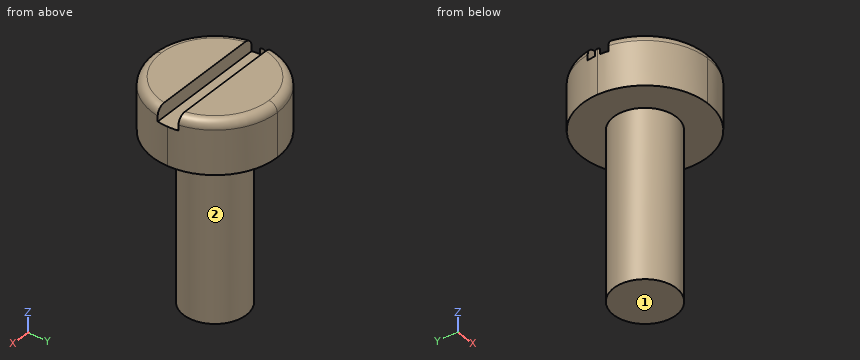
from build123d import *

# Parameters (mm, degrees)
F1_DEPTH    = 3.81
F2_T1_DEPTH = 22.225
F3_R        = 3.80999
F0_W        = 1.905
F0_H        = 10.16
F5_R        = 0.508
F7_DEPTH    = 0.8382


# Not quite as in the source:
# - a fillet or chamfer that OpenCascade refuses, or shapes differently, is made with other operations: its cross-section is extruded or revolved along the edge and cut away or added
# - a fillet or chamfer is up to 0.001 mm smaller than in the source, because OpenCascade refuses the exact size
# - ends of sketch curves that miss each other by under 0.0002 mm in the source are joined
# - a feature names something its author has since deleted; it is built from what else it names


with BuildPart() as f1:
    # F0 (on Front) → F1 (new body, symmetric)
    with BuildSketch(Plane.XZ):
        Polygon((-3.81, 3.175), (-3.81, 0), (-1.905, 0), (0, 0), (1.905, 0), (3.81, 0), (3.81, 3.175), align=None)
    extrude(amount=F1_DEPTH, both=True)

    # F2: fillet of radius 3.81 on 2 edges, made by hand

    # F2_s2 → F2_t1 (cut)
    with BuildSketch(Plane.XY.offset(-9.525)):
        with BuildLine():
            ThreePointArc((-3.81, 0), (-2.6940768363, -2.6940768363), (0, -3.81))
            Line((0, -3.81), (-3.81, -3.81))
            Line((-3.81, -3.81), (-3.81, 0))
        make_face()
        with BuildLine():
            ThreePointArc((-3.81, 0), (-2.6940768363, 2.6940768363), (0, 3.81))
            Line((0, 3.81), (-3.81, 3.81))
            Line((-3.81, 3.81), (-3.81, 0))
        make_face()
    extrude(amount=F2_T1_DEPTH, mode=Mode.SUBTRACT)

    # F3 (radius 3.81 in the source; OpenCascade refuses exactly that, so slightly less here)
    f3_edges = [f1.edges().sort_by_distance(p)[0] for p in [
        (3.81, -3.81, 1.5875),
        (3.81, 3.81, 1.5875),
    ]]
    fillet(f3_edges, radius=F3_R)

    # F0 (on Front) → F4 (revolve)
    with BuildSketch(Plane.XZ):
        with Locations((0.9525, -5.08)):
            Rectangle(F0_W, F0_H)
    revolve(axis=Axis((0, 0, -5.08), (0, 0, 1)))

    # F5
    f5_edges = [f1.edges().sort_by_distance(p)[0] for p in [
        (-2.694077, -2.694077, 3.175),
        (2.69408, -2.69408, 3.175),
        (5e-06, -3.81, 3.175),
        (-2.694077, 2.694077, 3.175),
        (2.69408, 2.69408, 3.175),
        (5e-06, 3.81, 3.175),
    ]]
    fillet(f5_edges, radius=F5_R)

    # F6 (on face) → F7 (cut)
    with BuildSketch(Plane.XY.offset(3.175)):
        with BuildLine():
            Line((-3.2403671088, 0.635), (-3.8071805373, 0.635))
            Line((-3.8071805373, 0.635), (-3.8071805373, -0.635))
            Line((-3.8071805373, -0.635), (-3.2403671088, -0.635))
            ThreePointArc((-3.2403671088, -0.635), (-3.2865556585, -0.3189920114), (-3.302, 0))
            ThreePointArc((-3.302, 0), (-3.2865556585, 0.3189920114), (-3.2403671088, 0.635))
        make_face()
        with BuildLine():
            Line((3.2403688783, 0.635), (-3.2403671088, 0.635))
            ThreePointArc((-3.2403671088, 0.635), (-3.2865556585, 0.3189920114), (-3.302, 0))
            ThreePointArc((-3.302, 0), (-3.2865556585, -0.3189920114), (-3.2403671088, -0.635))
            Line((-3.2403671088, -0.635), (3.2403688783, -0.635))
            ThreePointArc((3.2403688783, -0.635), (3.2865561029, -0.3189969493), (3.302, -1e-05))
            ThreePointArc((3.302, -1e-05), (3.2865561029, 0.3189969493), (3.2403688783, 0.635))
        make_face()
        with BuildLine():
            Line((3.8128194627, 0.635), (3.2403688783, 0.635))
            ThreePointArc((3.2403688783, 0.635), (3.2865561029, 0.3189969493), (3.302, 1e-05))
            ThreePointArc((3.302, 1e-05), (3.2865561029, -0.3189969493), (3.2403688783, -0.635))
            Line((3.2403688783, -0.635), (3.8128194627, -0.635))
            Line((3.8128194627, -0.635), (3.8128194627, 0.635))
        make_face()
    extrude(amount=-F7_DEPTH, mode=Mode.SUBTRACT)


solid = f1.part
Read the model definition and answer for the solid it produces. Units are mm, in the model's axes. Face numbers are marked on the shaded views. A direction names the side the tool comes from. Round coordinates to 2 decimals unless told otherwise and drop trailing zeros. Write each loop counter-clockwise with the first axis right and the second up, starting at its lowest first coordinate (ties: lowest second). Pieces come first, ordered by that corner, then holes. Notation, with made-up numbers: (89.25, 5) - (114.25, 5) arc R22 ccw to (114.25, 22) - close; hole circle Ø3 at (83.5, -30.5). An arc over 180 degrees is marked (long way). One line per question, with ' | ' between items. Start each with the question number.
1. For the marked faces 1 and 2, determine the directions among +Z, -Z, +X, -X, +Y, -Y from which every point of the face is accessible in a straight line to the end or side of a thin tool.
2. Find the intervals of material crossed by probe 1 along Z at (x, y) = (1.5, 0); probe 2 along Y at (x, z) = (0, -5) (3 decimals); probe 3 along Z at (x, y) = (-1.5, 3), in increasing order. Write a range as [from, to].
3. Each of these flat-tipped pins is pushed along its axis until it touches: pin 1 (0.6 mm diameter, centred on x = -1.5, y = 0, fed in from +Z); pin 2 (0.7 mm diameter, centred on x = 2, z = 3, fed in from -Y); pin 3 (3 mm diameter, centred on y = -1, z = 1.5, fed in from -X); pin 4 (1 mm diameter, centred on x = 1.5, z = -2.5, fed in from -Y). Where does it stop, or does it pass through?
4. Section A-A (z = -0.5) is taken. Determine the outline of the cut face in (x, y) (3 decimals).
Filled in:
1) face 1: -Z, +X, -X, +Y, -Y | face 2: -Z
2) probe 1: [-10.16, 2.34] | probe 2: [-1.905, 1.905] | probe 3: [0, 3.17]
3) pin 1: z = 2.34 | pin 2: y = -3.38 | pin 3: x = -3.81 | pin 4: y = -1.62
4) outline: circle Ø3.81 at (0, 0)
